Here's how the part is built. I have some questions about the finished solid (model axes, mm). Face numbers are marked on the shaded views. A direction names the side the tool comes from. Coordinates: 2 decimals unless noted, no trailing zeros. Loops run counter-clockwise (first coordinate to the right, second up) from the corner with the lowest first, then second, coordinate; pieces in that order, holes last. Notation, with made-up numbers: (78, -36.75) -> (116, -36.75) arc R23 ccw to (116, -24.75) -> close; hole circle Ø9 at (39, -25.75). An arc over 180 degrees is marked (long way). Answer as a JSON object with one key per item and string values. Group by question number.
Q1. On a 3-axis mill with a long thin cutter (end or side, diameter ignored), from which of +Z, -Z, +X, -X, +Y, -Y can I reach the whole of each face in a straight line? I mean the marked faces 1, 2 and 3. Say none if no direction works.
Q2. I want a section at C-C on z = 31.5. Write out the boundary of the cut face in (x, y) (3 decimals), then the cut area to 3 significant figures.
Q3. I want a section at A-A on y = 5. Write out the boundary of the cut face in (x, z).
Q4. I want a section at B-B on z = 12.75. Write out the boundary of the cut face in (x, y) (3 decimals), then the cut area to 3 significant figures.
Q5. I want a section at D-D on x = 21. Write out the boundary of the cut face in (y, z), then the cut area to 3 significant figures.
Q6. I'm going to push flat-ended pins straight in: pin 1 (3 mm diameter, centred on x = 29.845, z = -5.838, fed in from +Y); pin 2 (7 mm diameter, centred on y = 5, z = 50.088, fed in from -X); pin 3 (5 mm diameter, centred on x = 10, y = 6.5, fed in from -Z); pin 4 (6 mm diameter, centred on x = 12.5, y = 2.5, fed in from +Z). Where does each tip first touch, or does it pass through?
Q7. I need wall thicknesses on line 1 (X direction, y = 13, z = -7.5) (3 decimals); line 2 (X direction, y = 14, z = -7) (3 decimals); line 3 (Y direction, x = 31.5, z = 54). Which ranges of each line are inside material? Lowest first, please.
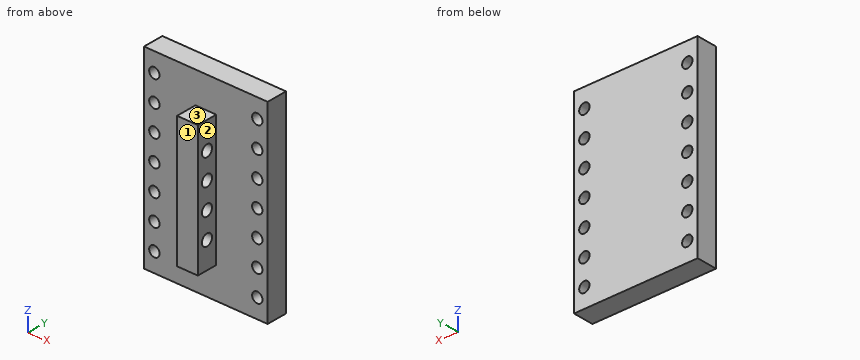
```python
from build123d import *

# Parameters (mm, degrees)
SKETCH1_W           = 10
SKETCH1_H           = 63
BOSS_EXTRUDE1_DEPTH = 10
SKETCH2_W           = 59.69
SKETCH2_H           = 93
SKETCH2_R           = 2.5
BOSS_EXTRUDE2_DEPTH = 10
SKETCH3_R           = 2.75
CUT_EXTRUDE1_DEPTH  = 88.739238799


with BuildPart() as part:
    # Sketch1 → Boss-Extrude1 (new body)
    with BuildSketch(Plane(origin=(0, 0, 0), x_dir=(1, 0, 0), z_dir=(0, 1, 0))):
        with Locations((5, -31.5)):
            Rectangle(SKETCH1_W, SKETCH1_H)
    extrude(amount=BOSS_EXTRUDE1_DEPTH)

    # Sketch2 → Boss-Extrude2 (add)
    with BuildSketch(Plane(origin=(0, 10, 0), x_dir=(1, 0, 0), z_dir=(0, 1, 0))):
        with Locations((5, -31.5)):
            Rectangle(SKETCH2_W, SKETCH2_H)
        with Locations(Location((-19.845, 5.838000036, 0), (0, 0, 270))):
            Circle(SKETCH2_R, mode=Mode.SUBTRACT)
        with Locations(Location((-19.845, -6.607999964, 0), (0, 0, 270))):
            Circle(SKETCH2_R, mode=Mode.SUBTRACT)
        with Locations(Location((-19.845, -19.053999964, 0), (0, 0, 270))):
            Circle(SKETCH2_R, mode=Mode.SUBTRACT)
        with Locations(Location((-19.845, -31.499999964, 0), (0, 0, 270))):
            Circle(SKETCH2_R, mode=Mode.SUBTRACT)
        with Locations(Location((-19.845, -43.945999964, 0), (0, 0, 270))):
            Circle(SKETCH2_R, mode=Mode.SUBTRACT)
        with Locations(Location((-19.845, -56.391999964, 0), (0, 0, 270))):
            Circle(SKETCH2_R, mode=Mode.SUBTRACT)
        with Locations(Location((-19.845, -68.837999964, 0), (0, 0, 270))):
            Circle(SKETCH2_R, mode=Mode.SUBTRACT)
        with Locations(Location((29.845, 5.838000036, 0), (0, 0, 270))):
            Circle(SKETCH2_R, mode=Mode.SUBTRACT)
        with Locations(Location((29.845, -6.607999964, 0), (0, 0, 270))):
            Circle(SKETCH2_R, mode=Mode.SUBTRACT)
        with Locations(Location((29.845, -19.053999964, 0), (0, 0, 270))):
            Circle(SKETCH2_R, mode=Mode.SUBTRACT)
        with Locations(Location((29.845, -31.499999964, 0), (0, 0, 270))):
            Circle(SKETCH2_R, mode=Mode.SUBTRACT)
        with Locations(Location((29.845, -43.945999964, 0), (0, 0, 270))):
            Circle(SKETCH2_R, mode=Mode.SUBTRACT)
        with Locations(Location((29.845, -56.391999964, 0), (0, 0, 270))):
            Circle(SKETCH2_R, mode=Mode.SUBTRACT)
        with Locations(Location((29.845, -68.837999964, 0), (0, 0, 270))):
            Circle(SKETCH2_R, mode=Mode.SUBTRACT)
    extrude(amount=BOSS_EXTRUDE2_DEPTH)

    # Sketch3 → Cut-Extrude1 (cut, through all)
    with BuildSketch(Plane.ZY):
        with Locations((12.75, 5)):
            Circle(SKETCH3_R)
        with Locations((25.196, 5)):
            Circle(SKETCH3_R)
        with Locations((37.642, 5)):
            Circle(SKETCH3_R)
        with Locations((50.088, 5)):
            Circle(SKETCH3_R)
    extrude(amount=-CUT_EXTRUDE1_DEPTH, mode=Mode.SUBTRACT)


solid = part.part
```
Result set:
{
 "1": {"face 1": "+Z, -Z, +X, -X, -Y", "face 2": "+Z, -Z, +X, -Y", "face 3": "+Z, +X, -X, -Y"},
 "2": {"outline": "(-24.845, 10) -> (-22.345, 10) -> (-22.345, 20) -> (-24.845, 20) -> close; (-17.345, 10) -> (0, 10) -> (0, 0) -> (10, 0) -> (10, 10) -> (27.345, 10) -> (27.345, 20) -> (-17.345, 20) -> close; (32.345, 10) -> (34.845, 10) -> (34.845, 20) -> (32.345, 20) -> close", "area": "597 mm²"},
 "3": {"outline": "(0, 0) -> (10, 0) -> (10, 10) -> (0, 10) -> close; (0, 15.5) -> (10, 15.5) -> (10, 22.45) -> (0, 22.45) -> close; (0, 27.95) -> (10, 27.95) -> (10, 34.89) -> (0, 34.89) -> close; (0, 40.39) -> (10, 40.39) -> (10, 47.34) -> (0, 47.34) -> close; (0, 52.84) -> (10, 52.84) -> (10, 63) -> (0, 63) -> close"},
 "4": {"outline": "(-24.845, 10) -> (0, 10) -> (0, 7.75) -> (10, 7.75) -> (10, 10) -> (34.845, 10) -> (34.845, 20) -> (-24.845, 20) -> close; (0, 0) -> (10, 0) -> (10, 2.25) -> (0, 2.25) -> close", "area": "642 mm²"},
 "5": {"outline": "(10, -15) -> (20, -15) -> (20, 78) -> (10, 78) -> close", "area": "930 mm²"},
 "6": {"pin 1": "passes through", "pin 2": "stops at x = 0", "pin 3": "stops at z = 0", "pin 4": "stops at z = 63"},
 "7": {"line 1": "x = -24.845 to -21.713, -17.977 to 27.977, 31.713 to 34.845", "line 2": "x = -24.845 to -22.059, -17.631 to 27.631, 32.059 to 34.845", "line 3": "y = 10 to 20"}
}
